Geometry check sheet. Reference: the model listing, model coordinates, mm. Face numbers are marked on the shaded views. Give positions to 0.01 mm unless a question says otherwise; leave off trailing zeros. Write each loop counter-clockwise with the first axis right and the second up, starting at its lowest first coordinate (ties: lowest second). Pieces come first, ordered by that corner, then holes.
(1) Cross-section at B-B (y = 29.5). Record the boundary of the cut face in (x, z).
(2) Thickness scan on line 1 along Z through (x, y) = (1, 101.5); line 2 along X through (y, z) = (10, 0); line 3 along X through (y, z) = (185, 0). Record the ranges inside material, lowest first.
(3) Cross-section at C-C (y = 175). Record the boundary of the cut face in (x, z), and give its area (3 significant figures).
(4) Depth check by flat-ended pin: P1, Ø8, axis at x = 5.5, z = 5, coming from the +Y side; P2, Ø3, axis at y = 90, z = 0.5, coming from the -X side; P3, Ø1.5, axis at x = -3.5, y = 19.5, coming from the +Z side; P4, Ø1.5, axis at x = -1.5, z = 10.5, coming from the -Y side. Enter the tip coordinate at first touch or a pass-through.
(5) Cross-section at A-A (z = 4). Record the boundary of the cut face in (x, y), and give its area (3 significant figures).
(6) Mould release check, pull along Z, two halves, no side actions. Record for the marked faces 1 and 2: +Z half, -Z half, draft (parallel to the pull), parting line (faces both ways), or undercut.
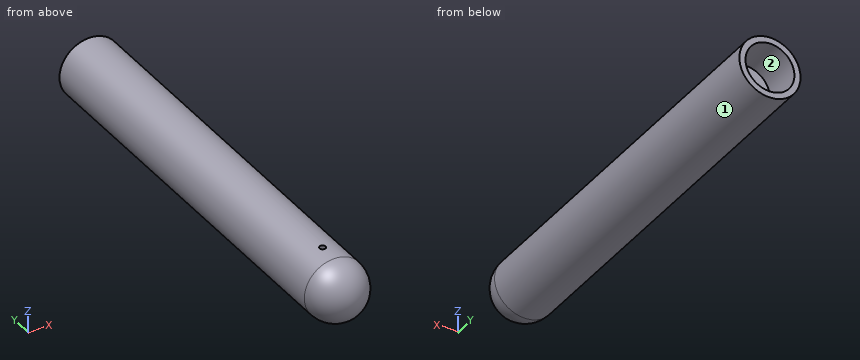
Autodesk Inventor part; units mm, degrees
ref_plane "YZ Plane" through (0, 0, 0) normal (1, 0, 0) x (0, 1, 0)
ref_plane "XZ Plane" through (0, 0, 0) normal (0, 1, 0) x (-1, 0, 0)
ref_plane "XY Plane" through (0, 0, 0) normal (0, 0, 1) x (1, 0, 0)
sketch "Sketch1" plane through (0, 0, 0) normal (0, 1, 0) x (-1, 0, 0)
  circle A0 centre (0, 0) radius 15
  circle A1 centre (0, 0) radius 12
  dimension "d0" = 30
  dimension "d1" = 3
extrude "Extrusion1" add sketch "Sketch1" along normal blind 200
sketch "Sketch2" plane through (0, 0, 0) normal (0, 0, 1) x (1, 0, 0)
  line L0 (0, 0) -> (15, 0)
  line L1 (15, 0) -> (15, -15)
  line L2 (15, -15) -> (0, -15)
  line L3 (0, -15) -> (0, 0)
  line L4 (15, 0) -> (-15, 0)
  circle A0 centre (0, 0) radius 15
  dimension "d4" = 15
  dimension "d5" = 15
revolve "Revolution1" add sketch "Sketch2" angle 360 about axis through (0, -15, 0) along (0, 1, 0) contours L0 A0 L3
sketch "Sketch3" plane through (0, 0, 0) normal (0, 0, 1) x (1, 0, 0)
  line L0 (0, 0) -> (0, 10)
  circle A0 centre (0, 10) radius 1.5
  circle A1 centre (0, 10) radius 2.5
  dimension "d7" = 10
  dimension "d8" = 3
  dimension "d9" = 5
extrude "Extrusion2" cut sketch "Sketch3" along normal blind 200 contours A0
extrude "Extrusion3" add sketch "Sketch3" against normal up to surface contours A0 | A1
extrude "Extrusion4" add sketch "Sketch3" along normal up to surface
extrude "Extrusion5" cut sketch "Sketch3" against normal blind 5.075 contours A0
sketch "Sketch4" plane through (0, 200, 0) normal (0, 1, 0) x (1, 0, 0)
  circle A0 centre (0, 0) radius 12
extrude "Extrusion6" add sketch "Sketch4" against normal blind 30
extrude "Extrusion7" cut sketch "Sketch4" against normal blind 20
properties part number "Tube_2"
Reply:
1. outline: circle Ø30 at (0, 0); hole circle Ø24 at (0, 0)
2. line 1: z = -14.97 to -11.96, 11.96 to 14.97
2. line 2: x = -15 to -12, -2.5 to -1.5, 1.5 to 2.5, 12 to 15
2. line 3: x = -15 to -12, 12 to 15
3. outline: circle Ø30 at (0, 0)
3. area: 707 mm2
4. P1: stops at y = 180
4. P2: stops at x = -15
4. P3: stops at z = 14.75
4. P4: stops at y = -11.31
5. outline: (-14.46, 0) arc R14.46 ccw to (14.46, 0) - (14.46, 200) - (11.31, 200) - (11.31, 180) - (-11.31, 180) - (-11.31, 200) - (-14.46, 200) - close; circle Ø5 at (0, 10); hole (-11.31, 0) - (11.31, 0) - (11.31, 170) - (-11.31, 170) - close; hole circle Ø3 at (0, 10)
5. area: 1,820 mm2
6. face 1: parting line
6. face 2: undercut
